The model under review builds one solid part; all positions refer to its coordinate system, in mm. Face numbers are marked on the shaded views. A direction names the side the tool comes from. Coordinates: 2 decimals unless noted, no trailing zeros. Write each loop counter-clockwise with the first axis right and the second up, starting at its lowest first coordinate (ties: lowest second). Pieces come first, ordered by that corner, then holes.
1) For line 1 (Z direction, x = 13.5, y = 6.3); line 2 (X direction, y = 16.6, z = 6); line 3 (Y direction, x = -1.5, z = 1.5), list the stretches that pass through material, from the lowest coordinate up.
2) Add section C-C, the plane x = 8. State the section outline as (y, z) points, then the cut area to 3 significant figures.
3) Add section A-A, the plane x = 13.5. State the section outline as (y, z) points.
4) For P1, Ø4, axis at y = -4, z = 8, coming from the +X side; P2, Ø6, axis at x = 13, z = 3, coming from the +Y side; P3, Ø1.8, axis at x = -8.5, z = 8.5, coming from the +Y side, all flat-tipped, find the tip position at first contact; note any pin that passes through.
5) Machinability: for the marked faces 1, 2, 3 and 4, which of the approach directions +Z, -Z, +X, -X, +Y, -Y give a long, thin tool a straight path to every point of the face, cutting with its end or side? Answer none if there is none.
6) Mouldability with a two-part tool opening along Z and no side actions: class the marked faces 5, 6, 7 and 8 as released by +Z, released by -Z, zero draft, split by the parting line, or undercut.
7) Add section B-B, the plane y = 9.5. State the section outline as (x, z) points, then the cut area to 3 significant figures.
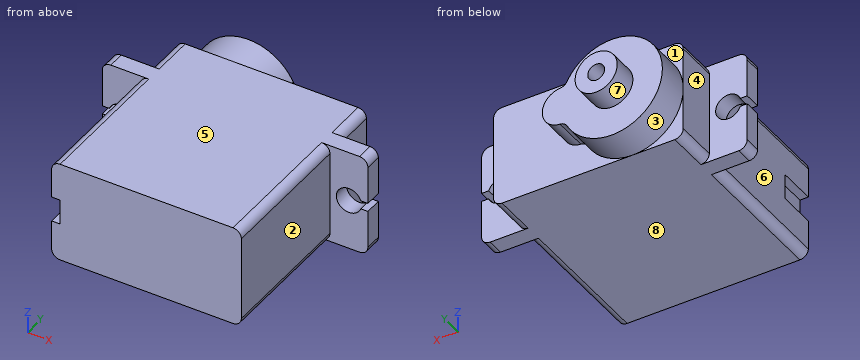
from build123d import *

# Parameters (mm, degrees)
EXTRUDE_1_DEPTH     = 12
EXTRUDE_2_DEPTH     = 4
CUT_EXTRUDE_1_DEPTH = 28.441984258
SKETCH_4_R          = 2.5
EXTRUDE_3_DEPTH     = 3
FILLET_1_R          = 1
FILLET_2_R          = 1
FILLET_3_R          = 1
SKETCH_5_R          = 1
CUT_EXTRUDE_2_DEPTH = 3
SKETCH_6_W          = 1
SKETCH_6_H          = 3
CUT_EXTRUDE_3_DEPTH = 4.5


with BuildPart() as part:
    # 草图1 → 凸台-拉伸1 (new body)
    with BuildSketch(Plane.XY):
        Polygon((-11.25, -12), (11.25, -12), (11.25, 5), (15.75, 5), (15.75, 7), (11.25, 7), (11.25, 12), (-11.25, 12), (-11.25, 7), (-15.75, 7), (-15.75, 5), (-11.25, 5), align=None)
    extrude(amount=EXTRUDE_1_DEPTH)

    # 草图2 → 凸台-拉伸2 (add)
    with BuildSketch(Plane(origin=(0, 12, 0), x_dir=(1, 0, 0), z_dir=(0, 1, 0))):
        with BuildLine():
            ThreePointArc((0.328125, -3.789904644), (-11.25, -6), (0.328125, -8.210095356))
            ThreePointArc((0.328125, -8.210095356), (3, -6), (0.328125, -3.789904644))
        make_face()
    extrude(amount=EXTRUDE_2_DEPTH)

    # 草图3 → 切除-拉伸1 (cut, through all)
    with BuildSketch(Plane(origin=(0, 7, 0), x_dir=(1, 0, 0), z_dir=(0, 1, 0))):
        with BuildLine():
            Line((15.75, -6.5), (14.914213562, -6.5))
            ThreePointArc((14.914213562, -6.5), (12, -6), (14.914213562, -5.5))
            Line((14.914213562, -5.5), (15.75, -5.5))
            Line((15.75, -5.5), (15.75, -6.5))
        make_face()
        with BuildLine():
            Line((-15.75, -5.5), (-14.914213562, -5.5))
            ThreePointArc((-14.914213562, -5.5), (-12, -6), (-14.914213562, -6.5))
            Line((-14.914213562, -6.5), (-15.75, -6.5))
            Line((-15.75, -6.5), (-15.75, -5.5))
        make_face()
    extrude(amount=-CUT_EXTRUDE_1_DEPTH, mode=Mode.SUBTRACT)

    # 草图4 → 凸台-拉伸3 (add)
    with BuildSketch(Plane(origin=(0, 16, 0), x_dir=(1, 0, 0), z_dir=(0, 1, 0))):
        with Locations(Location((-5.25, -6, 0), (0, 0, 270))):
            Circle(SKETCH_4_R)
    extrude(amount=EXTRUDE_3_DEPTH)

    # 圆角1
    fillet_1_edges = [part.edges().sort_by_distance(p)[0] for p in [
        (15.75, 6, 0),
        (-15.75, 6, 0),
        (-15.75, 6, 12),
        (15.75, 6, 12),
    ]]
    fillet(fillet_1_edges, radius=FILLET_1_R)

    # 圆角2
    fillet_2_edges = [part.edges().sort_by_distance(p)[0] for p in [
        (-11.25, 9.5, 12),
        (11.25, -3.5, 0),
        (-11.25, -3.5, 0),
        (-11.25, 9.5, 0),
        (11.25, 9.5, 0),
        (-11.25, -3.5, 12),
        (11.25, -3.5, 12),
        (11.25, 9.5, 12),
    ]]
    fillet(fillet_2_edges, radius=FILLET_2_R)

    # 圆角3
    fillet_3_edges = [part.edges().sort_by_distance(p)[0] for p in [
        (0.328125, 14, 8.210095356),
        (0.328125, 14, 3.789904644),
    ]]
    fillet(fillet_3_edges, radius=FILLET_3_R)

    # 草图5 → 切除-拉伸2 (cut)
    with BuildSketch(Plane(origin=(0, 19, 0), x_dir=(1, 0, 0), z_dir=(0, 1, 0))):
        with Locations(Location((-5.25, -6, 0), (0, 0, 270))):
            Circle(SKETCH_5_R)
    extrude(amount=-CUT_EXTRUDE_2_DEPTH, mode=Mode.SUBTRACT)

    # 草图6 → 切除-拉伸3 (cut)
    with BuildSketch(Plane.XZ.offset(12)):
        with Locations((-10.75, 6)):
            Rectangle(SKETCH_6_W, SKETCH_6_H)
    extrude(amount=-CUT_EXTRUDE_3_DEPTH, mode=Mode.SUBTRACT)


solid = part.part
Geometry results:
1. line 1: z = 0 to 4.5, 7.5 to 12
1. line 2: x = -7.75 to -6.25, -4.25 to -2.75
1. line 3: y = -12 to 16
2. outline: (-12, 0) - (12, 0) - (12, 12) - (-12, 12) - close
2. area: 288 mm2
3. outline: (5, 0) - (7, 0) - (7, 4.5) - (5, 4.5) - close; (5, 7.5) - (7, 7.5) - (7, 12) - (5, 12) - close
4. P1: stops at x = 11.25
4. P2: stops at y = 12
4. P3: stops at y = 16
5. face 1: +Z, -X, +Y
5. face 2: +Z, -Z, +X, -Y
5. face 3: +Y
5. face 4: +Z, -Z, -X, +Y
6. face 5: released by +Z
6. face 6: zero draft
6. face 7: split by the parting line
6. face 8: released by -Z
7. outline: (-11.25, 1) arc R1 ccw to (-10.25, 0) - (10.25, 0) arc R1 ccw to (11.25, 1) - (11.25, 11) arc R1 ccw to (10.25, 12) - (-10.25, 12) arc R1 ccw to (-11.25, 11) - close
7. area: 269 mm2
